from build123d import *

# Parameters (mm, degrees)
SKETCH1_R                = 8
BOSS_EXTRUDE1_DEPTH      = 25
BOSS_EXTRUDE2_DEPTH      = 240
BOSS_EXTRUDE3_REACH      = 252.402
BOSS_EXTRUDE3_END_RADIUS = 100
CUT_EXTRUDE1_START       = -45
CUT_EXTRUDE1_OUTLINE_R   = 8
CUT_EXTRUDE1_OUTLINE_R_2 = 10
CUT_EXTRUDE1_DEPTH       = 45
SKETCH4_R                = 3
CUT_EXTRUDE2_DEPTH       = 265.954713149


# Read off the part's stored shape, not the designer's step: Cut-Extrude1
with BuildPart() as part:
    # Sketch1 → Boss-Extrude1 (new body)
    with BuildSketch(Plane(origin=(0, 0, 0), x_dir=(1, 0, 0), z_dir=(0, 1, 0))):
        with BuildLine():
            Line((-15, 36), (-15, 25))
            Line((-15, 25), (-15, 23.5))
            Line((-15, 23.5), (15, 23.5))
            Line((15, 23.5), (15, 25))
            Line((15, 25), (15, 36))
            ThreePointArc((15, 36), (0, 51), (-15, 36))
        make_face()
        with Locations(Location((0, 36, 0), (0, 0, 270))):
            Circle(SKETCH1_R, mode=Mode.SUBTRACT)
    extrude(amount=-BOSS_EXTRUDE1_DEPTH)

    # Sketch1_3 → Boss-Extrude2 (add)
    with BuildSketch(Plane(origin=(0, 0, 0), x_dir=(1, 0, 0), z_dir=(0, 1, 0))):
        with BuildLine():
            Line((0, 23.5), (0, 10))
            ThreePointArc((0, 10), (25.88190451, 13.407417371), (50, 23.397459622))
            Line((50, 23.397459622), (50, 45))
            Line((50, 45), (25.673846837, 45))
            Line((25.673846837, 45), (35, 25))
            Line((35, 25), (15, 25))
            Line((15, 25), (15, 23.5))
            Line((15, 23.5), (0, 23.5))
        make_face()
        with BuildLine():
            Line((-50, 45), (-50, 23.397459622))
            ThreePointArc((-50, 23.397459622), (-25.88190451, 13.407417371), (0, 10))
            Line((0, 10), (0, 23.5))
            Line((0, 23.5), (-15, 23.5))
            Line((-15, 23.5), (-15, 25))
            Line((-15, 25), (-35, 25))
            Line((-35, 25), (-25.673846837, 45))
            Line((-25.673846837, 45), (-50, 45))
        make_face()
    extrude(amount=-BOSS_EXTRUDE2_DEPTH)

    # Boss-Extrude3: up to this cylinder (the profile starts outside it)
    boss_extrude3_end = Plane(origin=(0, -162.5, -110), z_dir=(0, 1, 0)) * Cylinder(BOSS_EXTRUDE3_END_RADIUS, 705.804, mode=Mode.PRIVATE)
    # Sketch2 → Boss-Extrude3 (add, up to the surface)
    with BuildSketch(Plane.XY, mode=Mode.PRIVATE) as boss_extrude3_sk1:
        with BuildLine():
            Line((50, -96.438424114), (50, -228.561575886))
            ThreePointArc((50, -228.561575886), (0, -240), (-50, -228.561575886))
            Line((-50, -228.561575886), (-50, -96.438424114))
            ThreePointArc((-50, -96.438424114), (0, -85), (50, -96.438424114))
        make_face()
    boss_extrude3_tool1 = extrude(boss_extrude3_sk1.sketch, amount=-BOSS_EXTRUDE3_REACH, mode=Mode.PRIVATE) - boss_extrude3_end
    add(boss_extrude3_tool1.solids().sort_by_distance((0, -162.5, 0))[0])

    # Cut-Extrude1 outline → Cut-Extrude1 (cut)
    with BuildSketch(Plane.XY.offset(CUT_EXTRUDE1_START)):
        with BuildLine():
            Line((2.37e-07, -240), (50, -240))
            Line((50, -240), (50, -228.561575886))
            ThreePointArc((50, -228.561575886), (25.645845521, -237.103927708), (2.37e-07, -240))
        make_face()
        with BuildLine():
            Line((-50, -228.561575886), (-50, -240))
            Line((-50, -240), (2.37e-07, -240))
            ThreePointArc((2.37e-07, -240), (-25.64584529, -237.103927761), (-50, -228.561575886))
        make_face()
        with Locations((0, -117)):
            Circle(CUT_EXTRUDE1_OUTLINE_R)
        with Locations((0, -205)):
            Circle(CUT_EXTRUDE1_OUTLINE_R_2)
    extrude(amount=CUT_EXTRUDE1_DEPTH, mode=Mode.SUBTRACT)

    # Sketch4 → Cut-Extrude2 (cut, through all)
    with BuildSketch(Plane(origin=(50, 0, 0), x_dir=(0, 0, -1), z_dir=(1, 0, 0))):
        with Locations((34.198729811, -63)):
            Circle(SKETCH4_R)
        with Locations((34.198729811, -113)):
            Circle(SKETCH4_R)
        with Locations((34.198729811, -163)):
            Circle(SKETCH4_R)
        with Locations((34.198729811, -213)):
            Circle(SKETCH4_R)
    extrude(amount=-CUT_EXTRUDE2_DEPTH, mode=Mode.SUBTRACT)


solid = part.part
Verification items for the finished model (mm, model axes). A direction names the side the tool comes from. Give positions to 0.01 mm unless a question says otherwise; leave off trailing zeros. Write each loop counter-clockwise with the first axis right and the second up, starting at its lowest first coordinate (ties: lowest second). Pieces come first, ordered by that corner, then holes. Notation, with made-up numbers: M 22.25,-28.75 L 51.25,-28.75 A33 ccw 51.25,1.25 Z; hole C 0.25,42 d5. An arc over 180 degrees is marked long. Use CSV: the item, a comma, the result in double quotes.
1) Access from +Z, -Z, +X, -X, +Y, -Y to the whole of each face (thin tool, end or side, straight path). Record for faces 5 (the face through (-39.51, -212.1, -37.06)), 6 (the face through (-0.724, -85.002, -6.336)), 7 (the face through (25, -118, -25)), 8 (the face through (15, -12, -30)).
Final values:
face 5,"+X, -X"
face 6,"+Z, +Y"
face 7,"+Y, -Y"
face 8,"-Z, +Y, -Y"
2) Cross-section at A-A (y = -205). Enter the section's corners in (x, z), plus the area to 3 significant figures.
Final values:
outline,"M -50,-45 L -25.67,-45 L -35,-25 L -15,-25 L -15,-23.5 L -10,-23.5 L -10,0 L -50,0 Z; M 10,-23.5 L 15,-23.5 L 15,-25 L 35,-25 L 25.67,-45 L 50,-45 L 50,0 L 10,0 Z"
area,"2,770 mm²"
3) Go/stop test with flat-tipped pins: pin 1 Ø3 at (y, z) = (-67, -45.5) entering from +X; pin 2 Ø1.5 at (x, y) = (-5.5, -167.5) entering from -Z; pin 3 Ø8 at (x, z) = (-4.5, -40.5) entering from -Y; pin 4 Ø1.5 at (x, z) = (-37, -13) entering from +Y. Record where each tip stops, or that it passes through.
Final values:
pin 1,"x = 50"
pin 2,"z = -23.5"
pin 3,"y = -25"
pin 4,"y = -90.86"
4) Cross-section at C-C (y = -63). Enter the section's corners in (x, z), plus the area to 3 significant figures.
Final values:
outline,"M -50,-45 L -25.67,-45 L -29.31,-37.2 L -50,-37.2 Z; M -50,-31.2 L -32.11,-31.2 L -35,-25 L -15,-25 L -15,-23.5 L 15,-23.5 L 15,-25 L 35,-25 L 32.11,-31.2 L 50,-31.2 L 50,-23.4 A100 ccw -50,-23.4 Z; M 25.67,-45 L 50,-45 L 50,-37.2 L 29.31,-37.2 Z"
area,"1,580 mm²"
5) Material ranges on line 1 along Y through (x, z) = (0, -14.25); line 2 along Z through (x, y) = (34.25, -163); line 3 along Y through (x, z) = (41, -35), recorded low to high.
Final values:
line 1,"-240 to -215, -195 to -125, -109 to 0"
line 2,"-45 to -37.2, -31.2 to -26.61, -25 to 0"
line 3,"-232.44 to -215.89, -210.11 to -165.89, -160.11 to -115.89, -110.11 to -65.89, -60.11 to 0"
6) Release check for a two-part mould opening along Y. For faces 1 (the face through (-39.51, -162.1, -37.06)), 2 (the face through (-6.9, -25, -40.5)), 3 (the face through (39.8, -62.1, -37.06)), 4 (the face through (-15, -12, -31)) record: released by +Y, released by -Y, zero draft, split by the parting line, or undercut.
Final values:
face 1,"undercut"
face 2,"released by -Y"
face 3,"undercut"
face 4,"zero draft"
7) Cross-section at B-B (x = -4). Enter the section's corners in (y, z), plus the area to 3 significant figures.
Final values:
outline,"M -239.93,-23.5 L -214.17,-23.5 L -214.17,0 L -239.93,0 Z; M -195.83,-23.5 L -123.93,-23.5 L -123.93,0 L -195.83,0 Z; M -110.07,-23.5 L -25,-23.5 L -25,-29.07 L 0,-29.07 L 0,-10.08 L -85.07,-10.08 L -85.07,0 L -110.07,0 Z; M -25,-50.46 L 0,-50.46 L 0,-42.93 L -25,-42.93 Z"
area,"4,350 mm²"
8) Cross-section at D-D (z = -17). Enter the section's corners in (x, y).
Final values:
outline,"M -50,-228.56 A115 ccw 50,-228.56 L 50,-96.44 A115 ccw 36.76,-91.03 L 36.76,0 L -36.76,0 L -36.76,-91.03 A115 ccw -50,-96.44 Z; hole C 0,-205 d20; hole C 0,-117 d16"
